Can you work these out from the model? Positions are in its coordinate system, mm. A direction names the side the tool comes from. Give positions to 0.01 mm unless a question says otherwise; leave off trailing zeros. Order: outer loops, then holes, each group sorted by start corner. A loop starts at its lowest first (then second) coordinate and runs counter-clockwise, first axis right, second up.
Item 1: I'm going to push flat-ended pins straight in: pin 1 Ø5 at (x, z) = (-11.5, 163.5) entering from +Y; pin 2 Ø1.5 at (y, z) = (5.5, 85) entering from -X; pin 3 Ø3 at (x, y) = (1.5, -6.5) entering from +Z. Where does each tip first touch, or does it pass through?
Item 2: Which directions (+Z, -Z, +X, -X, +Y, -Y) give clear straight access to the entire face, cutting with the end or side of a thin tool? Please do faces 5 (the cylindrical face through (-11.99, 0.53, 186.65)), 6 (the flat face through (0, 0, 227)), 7 (the flat face through (-11, 17, 3)).
Item 3: I want a section at D-D, the plane z = 121. Write out the boundary of the cut face in (x, y).
Item 4: I want a section at A-A, the plane y = 15.5. Write out the boundary of the cut face in (x, z), then the cut area to 3 significant figures.
Item 5: I want a section at C-C, the plane z = 182. Write out the boundary of the cut face in (x, y).
Item 6: If I drill on line 1 along Z through (x, y) = (16, 13.5); line 2 along Z through (x, y) = (-12, -3); line 3 along X through (y, z) = (1, 154), over which ranges is the centre line in solid material (lowest first)?
Item 7: If we mould it in two halves opening along Z, with no side actions, what happens to faces 1 (the flat face through (-6, -11, 56)), 2 (the flat face through (-6, -11, 162)), 3 (the flat face through (-11, 17, 53)), 4 (the cylindrical face through (23.846, 7.509, 1.479))? For each: +Z half, -Z half, draft (parallel to the pull), parting line (faces both ways), or undercut.
```python
from build123d import *

# Parameters (mm, degrees)
SKETCH_1_R      = 25
EXTRUDE_1_DEPTH = 3
SKETCH_2_R      = 20
EXTRUDE_2_DEPTH = 50
SKETCH_3_R      = 25
EXTRUDE_3_DEPTH = 3
SKETCH_4_R      = 12
EXTRUDE_4_DEPTH = 50
SKETCH_5_R      = 25
EXTRUDE_5_DEPTH = 3
SKETCH_6_R      = 20
EXTRUDE_6_DEPTH = 50
SKETCH_8_R      = 25
EXTRUDE_7_DEPTH = 3
SKETCH_9_R      = 12
EXTRUDE_8_DEPTH = 50
SKETCH_10_R     = 5
EXTRUDE_9_DEPTH = 15


with BuildPart() as part:
    # 草图1 → 凸台-拉伸1 (new body)
    with BuildSketch(Plane.XY):
        Circle(SKETCH_1_R)
    extrude(amount=EXTRUDE_1_DEPTH)

    # 草图2 → 凸台-拉伸2 (add)
    with BuildSketch(Plane.XY.offset(3)):
        Circle(SKETCH_2_R)
    extrude(amount=EXTRUDE_2_DEPTH)

    # 草图3 → 凸台-拉伸3 (add)
    with BuildSketch(Plane.XY.offset(53)):
        Circle(SKETCH_3_R)
    extrude(amount=EXTRUDE_3_DEPTH)

    # 草图4 → 凸台-拉伸4 (add)
    with BuildSketch(Plane.XY.offset(56)):
        Circle(SKETCH_4_R)
    extrude(amount=EXTRUDE_4_DEPTH)

    # 草图5 → 凸台-拉伸5 (add)
    with BuildSketch(Plane.XY.offset(106)):
        Circle(SKETCH_5_R)
    extrude(amount=EXTRUDE_5_DEPTH)

    # 草图6 → 凸台-拉伸6 (add)
    with BuildSketch(Plane.XY.offset(109)):
        Circle(SKETCH_6_R)
    extrude(amount=EXTRUDE_6_DEPTH)

    # 草图8 → 凸台-拉伸7 (add)
    with BuildSketch(Plane.XY.offset(159)):
        Circle(SKETCH_8_R)
    extrude(amount=EXTRUDE_7_DEPTH)

    # 草图9 → 凸台-拉伸8 (add)
    with BuildSketch(Plane.XY.offset(162)):
        Circle(SKETCH_9_R)
    extrude(amount=EXTRUDE_8_DEPTH)

    # 草图10 → 凸台-拉伸9 (add)
    with BuildSketch(Plane.XY.offset(212)):
        Circle(SKETCH_10_R)
    extrude(amount=EXTRUDE_9_DEPTH)


solid = part.part
```
Results list:
1. pin 1: stops at y = 23.12
1. pin 2: stops at x = -11.02
1. pin 3: stops at z = 212
2. face 5: +Z
2. face 6: +Z, +X, -X, +Y, -Y
2. face 7: none
3. outline: circle Ø40 at (0, 0)
4. outline: (-19.62, 0) - (19.62, 0) - (19.62, 3) - (12.64, 3) - (12.64, 53) - (19.62, 53) - (19.62, 56) - (-19.62, 56) - (-19.62, 53) - (-12.64, 53) - (-12.64, 3) - (-19.62, 3) - close; (-19.62, 106) - (19.62, 106) - (19.62, 109) - (12.64, 109) - (12.64, 159) - (19.62, 159) - (19.62, 162) - (-19.62, 162) - (-19.62, 159) - (-12.64, 159) - (-12.64, 109) - (-19.62, 109) - close
4. area: 3,000 mm2
5. outline: circle Ø24 at (0, 0)
6. line 1: z = 0 to 3, 53 to 56, 106 to 109, 159 to 162
6. line 2: z = 0 to 56, 106 to 162
6. line 3: x = -19.97 to 19.97
7. face 1: undercut
7. face 2: +Z half
7. face 3: undercut
7. face 4: draft
